```python
from build123d import *

# Parameters (mm, degrees)
SKETCH1_R           = 11.25
BOSS_EXTRUDE1_DEPTH = 60
SKETCH6_R           = 2.15
CUT_EXTRUDE5_DEPTH  = 77.321687612
CUT_EXTRUDE6_START  = -25
CUT_EXTRUDE6_DEPTH  = 25
FILLET3_R           = 2
CUT_EXTRUDE7_DEPTH  = 79.102496759
FILLET5_R           = 5
SKETCH9_R           = 20.5
CUT_EXTRUDE8_DEPTH  = 8
SKETCH10_R          = 11.25
BOSS_EXTRUDE2_DEPTH = 8
SKETCH12_R          = 1.65
CUT_EXTRUDE9_DEPTH  = 14
FILLET7_R           = 5
FILLET8_R           = 3


with BuildPart() as part:
    # Sketch1 → Boss-Extrude1 (new body)
    with BuildSketch(Plane.XY):
        with BuildLine():
            Line((-40, 15.05), (40, 15.05))
            Line((40, 15.05), (40, 10.05))
            Line((40, 10.05), (14.933100817, 10.05))
            ThreePointArc((14.933100817, 10.05), (17.662807084, -3.467743633), (10.024844138, -14.95))
            Line((10.024844138, -14.95), (-10.024844138, -14.95))
            ThreePointArc((-10.024844138, -14.95), (-17.662807084, -3.467743633), (-14.933100817, 10.05))
            Line((-14.933100817, 10.05), (-40, 10.05))
            Line((-40, 10.05), (-40, 15.05))
        make_face()
        with Locations(Location((0, 0, 0), (0, 0, 180))):
            Circle(SKETCH1_R, mode=Mode.SUBTRACT)
    extrude(amount=BOSS_EXTRUDE1_DEPTH)

    # Sketch6 → Cut-Extrude5 (cut, through all)
    with BuildSketch(Plane(origin=(0, 10.05, 0), x_dir=(-1, 0, 0), z_dir=(0, -1, 0))):
        with Locations(Location((33, -53, 0), (0, 0, 90))):
            Circle(SKETCH6_R)
        with Locations(Location((33, -7, 0), (0, 0, 90))):
            Circle(SKETCH6_R)
        with Locations(Location((-33, -53, 0), (0, 0, 90))):
            Circle(SKETCH6_R)
        with Locations(Location((-33, -7, 0), (0, 0, 90))):
            Circle(SKETCH6_R)
    extrude(amount=-CUT_EXTRUDE5_DEPTH, mode=Mode.SUBTRACT)

    # Sketch7 → Cut-Extrude6 (cut)
    with BuildSketch(Plane.XY.offset(60).offset(CUT_EXTRUDE6_START)):
        with BuildLine():
            Line((-14.933100817, 10.05), (14.933100817, 10.05))
            ThreePointArc((14.933100817, 10.05), (0, -18), (-14.933100817, 10.05))
        make_face()
    extrude(amount=CUT_EXTRUDE6_DEPTH, mode=Mode.SUBTRACT)

    # Fillet3
    fillet3_edges = [part.edges().sort_by_distance(p)[0] for p in [
        (-40, 12.55, 0),
        (40, 12.55, 60),
        (-40, 12.55, 60),
        (40, 12.55, 0),
    ]]
    fillet(fillet3_edges, radius=FILLET3_R)

    # Sketch8 → Cut-Extrude7 (cut, through all)
    with BuildSketch(Plane(origin=(0, 15.05, 0), x_dir=(1, 0, 0), z_dir=(0, 1, 0))):
        Polygon((0, -52), (8, -60), (-8, -60), align=None)
    extrude(amount=-CUT_EXTRUDE7_DEPTH, mode=Mode.SUBTRACT)

    # Fillet5
    fillet5_edges = [part.edges().sort_by_distance(p)[0] for p in [
        (-8, 12.55, 60),
        (8, 12.55, 60),
    ]]
    fillet(fillet5_edges, radius=FILLET5_R)

    # Sketch9 → Cut-Extrude8 (cut)
    with BuildSketch(Plane(origin=(0, 0, 0), x_dir=(-1, 0, 0), z_dir=(0, 0, -1))):
        Circle(SKETCH9_R)
    extrude(amount=-CUT_EXTRUDE8_DEPTH, mode=Mode.SUBTRACT)

    # Sketch10 → Boss-Extrude2 (add)
    with BuildSketch(Plane(origin=(0, 0, 8), x_dir=(-1, 0, 0), z_dir=(0, 0, -1))):
        with BuildLine():
            Line((-13.919321104, 15.05), (13.919321104, 15.05))
            ThreePointArc((13.919321104, 15.05), (20.499868756, 0.073355309), (14.026671023, -14.95))
            Line((14.026671023, -14.95), (-14.026671023, -14.95))
            ThreePointArc((-14.026671023, -14.95), (-20.499868756, 0.073355309), (-13.919321104, 15.05))
        make_face()
        Circle(SKETCH10_R, mode=Mode.SUBTRACT)
    extrude(amount=-BOSS_EXTRUDE2_DEPTH)

    # Sketch12 → Cut-Extrude9 (cut)
    with BuildSketch(Plane(origin=(0, 0, 8), x_dir=(-1, 0, 0), z_dir=(0, 0, -1))):
        with Locations((-16, 0)):
            Circle(SKETCH12_R)
        with Locations((-11.313708499, 11.313708499)):
            Circle(SKETCH12_R)
        with Locations((-11.313708499, -11.313708499)):
            Circle(SKETCH12_R)
        with Locations((11.313708499, -11.313708499)):
            Circle(SKETCH12_R)
        with Locations((16, 0)):
            Circle(SKETCH12_R)
        with Locations((11.313708499, 11.313708499)):
            Circle(SKETCH12_R)
    extrude(amount=-CUT_EXTRUDE9_DEPTH, mode=Mode.SUBTRACT)

    # Fillet7
    fillet7_edges = [part.edges().sort_by_distance(p)[0] for p in [
        (-17.867498426, 10.05, 12),
        (17.867498426, 10.05, 12),
    ]]
    fillet(fillet7_edges, radius=FILLET7_R)

    # Fillet8
    fillet8_edges = [part.edges().sort_by_distance(p)[0] for p in [
        (14.933100817, 10.05, 25.5),
        (-14.933100817, 10.05, 25.5),
    ]]
    fillet(fillet8_edges, radius=FILLET8_R)


solid = part.part
```
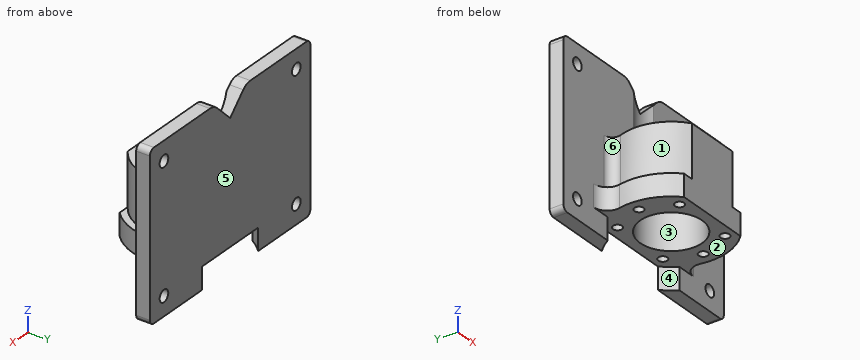
Can you work these out from the model? Positions are in its coordinate system, mm. Face numbers are marked on the shaded views. A direction names the side the tool comes from. Give positions to 0.01 mm unless a question says otherwise; leave off trailing zeros. Loops run counter-clockwise (first coordinate to the right, second up) from the corner with the lowest first, then second, coordinate; pieces in that order, holes last. Notation, with made-up numbers: M 54,55 L 87,55 A13 ccw 87,65 Z; hole C -26,-8.75 d2. An arc over 180 degrees is marked long. Answer in a Markdown table with one row per item.
1. Suppose I cut it at C-C on y = 3. Write out the boundary of the cut face in (x, z), plus the area to 3 significant figures.
Taken from the geometry:
| item | result |
|---|---|
| outline | M -20.28,8 L -10.84,8 L -10.84,35 L -17.75,35 L -17.75,16 L -20.28,16 Z; M 10.84,8 L 20.28,8 L 20.28,16 L 17.75,16 L 17.75,35 L 10.84,35 Z |
| area | 413 mm² |
2. Suppose I cut it at A-A on x = 33. Write out the boundary of the cut face in (y, z).
Taken from the geometry:
| item | result |
|---|---|
| outline | M 10.05,0 L 15.05,0 L 15.05,4.85 L 10.05,4.85 Z; M 10.05,9.15 L 15.05,9.15 L 15.05,50.85 L 10.05,50.85 Z; M 10.05,55.15 L 15.05,55.15 L 15.05,60 L 10.05,60 Z |
3. Suppose I cut it at D-D on z = 19. Write out the boundary of the cut face in (x, y), plus the area to 3 significant figures.
Taken from the geometry:
| item | result |
|---|---|
| outline | M -40,10.05 L -19.78,10.05 A3 cw -16.96,6.04 A18 ccw -10.02,-14.95 L 10.02,-14.95 A18 ccw 16.96,6.04 A3 cw 19.78,10.05 L 40,10.05 L 40,15.05 L -40,15.05 Z; hole C -16,0 d3.3; hole C -11.31,-11.31 d3.3; hole C -11.31,11.31 d3.3; hole C 0,0 d22.5; hole C 11.31,-11.31 d3.3; hole C 11.31,11.31 d3.3; hole C 16,0 d3.3 |
| area | 770 mm² |
4. Which directions (+Z, -Z, +X, -X, +Y, -Y) give clear straight access to the entire face, cutting with the end or side of a thin tool? Please do the marked faces 1, 2 and 3.
Taken from the geometry:
| item | result |
|---|---|
| face 1 | +Z, -X |
| face 2 | -Z, -Y |
| face 3 | +Z, -Z |
5. If I drill on line 1 along Y through (x, z) = (25, 28); line 2 along X through (y, z) = (5.5, 13); line 3 along X through (y, z) = (-5.5, 26.5), over which ranges is the centre line in solid material (lowest first)?
Taken from the geometry:
| item | result |
|---|---|
| line 1 | y = 10.05 to 15.05 |
| line 2 | x = -20.02 to -9.81, 9.81 to 20.02 |
| line 3 | x = -17.14 to -9.81, 9.81 to 17.14 |
6. Suppose I cut it at B-B on z = 7. Write out the boundary of the cut face in (x, y).
Taken from the geometry:
| item | result |
|---|---|
| outline | M -40,10.05 L -35.15,10.05 L -35.15,15.05 L -40,15.05 Z; M -30.85,10.05 L -17.87,10.05 A20.5 cw -13.92,15.05 L -30.85,15.05 Z; M 13.92,15.05 A20.5 cw 17.87,10.05 L 30.85,10.05 L 30.85,15.05 Z; M 35.15,10.05 L 40,10.05 L 40,15.05 L 35.15,15.05 Z |
7. For pin 1 Ø6 at (y, z) = (5, 15.5) entering from +X; pin 2 Ø10.5 at (x, z) = (-21.5, 40.5) entering from -Y; pin 3 Ø4 at (x, y) = (-16, 0) entering from +Z, each with a flat end and sliding along its axis, tell me the tip position at first contact or that it passes through.
Taken from the geometry:
| item | result |
|---|---|
| pin 1 | stops at x = 20.96 |
| pin 2 | stops at y = 10.05 |
| pin 3 | stops at z = 35 |
8. Thinking about a two-plate mould opening in Y: for the marked faces 4, 5 and 6, which applies, released by +Y, released by -Y, zero draft, split by the parting line, or undercut?
Taken from the geometry:
| item | result |
|---|---|
| face 4 | released by -Y |
| face 5 | released by +Y |
| face 6 | undercut |
